Work out the finished part from the listing and answer in its coordinate system (mm). A direction names the side the tool comes from. Coordinates: 2 decimals unless noted, no trailing zeros. Write each loop counter-clockwise with the first axis right and the second up, starting at its lowest first coordinate (ties: lowest second). Pieces come first, ordered by that corner, then holes. Notation, with made-up numbers: (55.5, 2) - (100.5, 2) arc R25 ccw to (100.5, 33) - close; hole circle Ø1 at (8, -34.75). An arc over 180 degrees is marked (long way). Use a Markdown table: item, result. Add a question column.
(1) The part is cut by section D-D, the plane y = 5.75. Give the vertices of the cut face in (x, z), then the cut area to 3 significant figures.
(2) The part is cut by section B-B, the plane z = 2.3. Give the vertices of the cut face in (x, y).
(3) Given pin 1 Ø2.5 at (x, y) = (0, 0) entering from -Z; pin 2 Ø3 at (x, y) = (1, -1) entering from -Z; pin 3 Ø2 at (y, z) = (-4, 3) entering from +X, each flat-ended and moving along its own axis, determine where each tip first touches the part or whether it passes through.
(4) The part is cut by section C-C, the plane y = -5. Give the vertices of the cut face in (x, z), then the cut area to 3 significant figures.
(5) A tool of negligible diameter and unlimited length cuts with its end or side. For faces 1 (the face through (-61, 0, 6)), 2 (the face through (1.3, -1.3, 3.25)), from which of +Z, -Z, +X, -X, +Y, -Y can it reach the whole face along a straight path? Write none if from no direction.
(6) The part is cut by section A-A, the plane y = 0. Give the vertices of the cut face in (x, z), then the cut area to 3 significant figures.
(7) Find the intervals of material crossed by line 1 (Y direction, x = 0, z = 4.65); line 2 (Y direction, x = 0, z = 2.25); line 3 (X direction, y = -0.25, z = 0.35), in increasing order. Write a range as from..to.
(8) For a pull along Y with two mould halves and no side action, classify faces 3 (the face through (-1.27, 0.97, 4.61)), 4 (the face through (-59, 10, 3)), 5 (the face through (-59, -10, 3)) as released by +Y, released by -Y, zero draft, split by the parting line, or undercut.
Autodesk Fusion 360 part; units mm, degrees
sketch "Sketch4" plane through (0, 0, 0) normal (0, 0, 1) x (1, 0, 0)
  circle A0 centre (0, 0) radius 3
  circle A1 centre (0, 0) radius 6
  dimension "d9" = 6
  dimension "d10" = 3
extrude "Extrude2" add sketch "Sketch4" along normal blind 3.25
sketch "Sketch5" plane through (0, 0, 3.25) normal (0, 0, 1) x (1, 0, 0)
  circle A0 centre (0, 0) radius 3
  circle A1 centre (0, 0) radius 6
  circle A2 centre (0, 0) radius 1.6
  dimension "d13" = 3.2
extrude "Extrude3" add sketch "Sketch5" along normal blind 2.75 contours A0 | A1
sketch "Sketch8" plane through (0, 0, 6) normal (0, 0, 1) x (1, 0, 0)
  circle A0 centre (0, 0) radius 1.6
  circle A1 centre (0, 0) radius 6
  circle A2 centre (0, 0) radius 10
  line L0 (0, -10) -> (0, 10) construction
  line L1 (0, -10) -> (-120, -10)
  line L2 (0, 10) -> (-120, 10)
  circle A3 centre (-120, 0) radius 10
  line L3 (-120, -10) -> (-120, 10) construction
  dimension "d30" = 20
  dimension "d31" = 120
  dimension "d32" = 120
extrude "Extrude5" add sketch "Sketch8" against normal up to surface (6 mm away) contours A2 | A2 L1 L2 A3 | A3
Model answer:
| question | item | result |
|---|---|---|
| 1 | outline | (-128.18, 0) - (8.18, 0) - (8.18, 6) - (-128.18, 6) - close |
| 1 | area | 818 mm^2 |
| 2 | outline | (-120, -10) - (0, -10) arc R10 ccw to (0, 10) - (-120, 10) arc R10 ccw to start; hole circle Ø6 at (0, 0) |
| 3 | pin 1 | through |
| 3 | pin 2 | z = 3.25 |
| 3 | pin 3 | x = 9.54 |
| 4 | outline | (-128.66, 0) - (8.66, 0) - (8.66, 6) - (-128.66, 6) - close |
| 4 | area | 824 mm^2 |
| 5 | face 1 | +Z, +X, -X, +Y, -Y |
| 5 | face 2 | -Z |
| 6 | outline | (-130, 0) - (-3, 0) - (-3, 3.25) - (-1.6, 3.25) - (-1.6, 6) - (-130, 6) - close; (1.6, 3.25) - (3, 3.25) - (3, 0) - (10, 0) - (10, 6) - (1.6, 6) - close |
| 6 | area | 812 mm^2 |
| 7 | line 1 | -10..-1.6, 1.6..10 |
| 7 | line 2 | -10..-3, 3..10 |
| 7 | line 3 | -130..-2.99, 2.99..10 |
| 8 | face 3 | undercut |
| 8 | face 4 | released by +Y |
| 8 | face 5 | released by -Y |
